Can you work these out from the model? Positions are in its coordinate system, mm. Face numbers are marked on the shaded views. A direction names the side the tool comes from. Coordinates: 2 decimals unless noted, no trailing zeros. Order: outer loops, then holes, each group sorted by start corner. A loop starts at its lowest first (then second) coordinate and runs counter-clockwise, first axis right, second up. Notation, with made-up numbers: (-11, -14) -> (25, -14) arc R17 ccw to (25, -4) -> close; hole circle Ø1 at (-31.75, 55). An arc over 180 degrees is marked (long way). Use a Markdown table: item, result. Add a question column.
1. For pin 1 Ø1.5 at (y, z) = (16.5, 2.5) entering from +X; pin 2 Ø6 at (x, z) = (2, -1) entering from -Y; pin 3 Ø2 at (x, y) = (5.5, 5.5) entering from -Z; pin 4 Ø1.6 at (x, y) = (0, 17.5) entering from -Z, each with a flat end and sliding along its axis, tell me the tip position at first contact or that it passes through.
2. Suppose I cut it at D-D, the plane y = 12.75. List the corners of the cut face in (x, z) for me, then the cut area to 3 significant figures.
3. For the marked faces 4 and 5, which set-ups out of +Z, -Z, +X, -X, +Y, -Y let a thin tool reach every point of the face, with its end or its side?
4. We'd pull the mould along Z, two halves only. Please class the marked faces 1, 2 and 3: pulls with the +Z half, pulls with the -Z half, needs draft (parallel to the pull), parting line crosses it, or undercut.
5. Suppose I cut it at B-B, the plane x = 0. List the corners of the cut face in (y, z) for me.
6. If I drill on line 1 along Z through (x, y) = (0, 4.1); line 2 along X through (y, z) = (17, 0); line 3 along X through (y, z) = (2.75, -0.25), over which ranges is the centre line in solid material (lowest first)? Write a range as from..to.
7. Suppose I cut it at C-C, the plane x = 5.75. List the corners of the cut face in (y, z) for me, then the cut area to 3 significant figures.
8. Suppose I cut it at A-A, the plane y = 3. List the corners of the cut face in (x, z) for me, then the cut area to 3 significant figures.
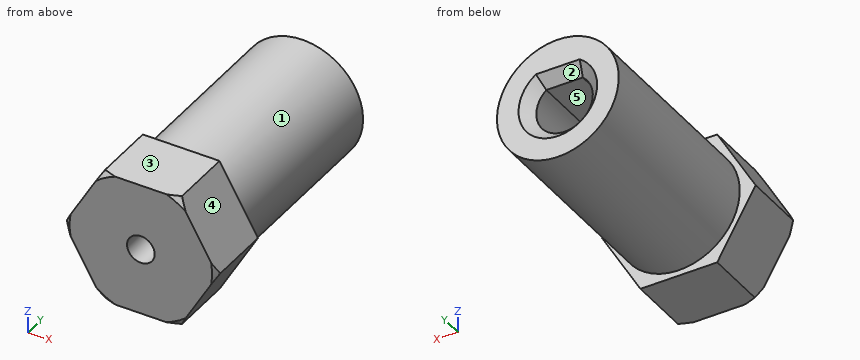
Autodesk Inventor part; units mm, degrees
ref_plane "YZ Plane" through (0, 0, 0) normal (1, 0, 0) x (0, 1, 0)
ref_plane "XZ Plane" through (0, 0, 0) normal (0, 1, 0) x (-1, 0, 0)
ref_plane "XY Plane" through (0, 0, 0) normal (0, 0, 1) x (1, 0, 0)
sketch "Sketch7" plane through (0, 0, 0) normal (0, 1, 0) x (-1, 0, 0)
  line L0 (-3.4641, -6) -> (-6.9282, 0)
  line L1 (-6.9282, 0) -> (-3.4641, 6)
  line L2 (-3.4641, 6) -> (3.4641, 6)
  line L3 (3.4641, 6) -> (6.9282, 0)
  line L4 (6.9282, 0) -> (3.4641, -6)
  line L5 (3.4641, -6) -> (-3.4641, -6)
  point P0 (0, 0)
  point P1 (0, 0)
  point P2 (0, -6)
  dimension "d24" = 12
extrude "Extrusion6" add sketch "Sketch7" along normal blind 6
sketch "Sketch8" plane through (0, 6, 0) normal (0, 1, 0) x (1, 0, 0)
  circle A0 centre (0, 0) radius 5.5
  circle A1 centre (0, 0) radius 2.55
  line L0 (-0.0689, 2.5491) -> (-0.0689, -1.9509)
  line L1 (-0.0689, -1.9509) -> (-1.6421, -1.9509)
  line L2 (-0.0689, -1.9509) -> (1.6421, -1.9509)
  dimension "d27" = 11
  dimension "d28" = 5.1
  dimension "d29" = 4.5
  dimension "d30" = 1.5732
extrude "Extrusion7" add sketch "Sketch8" along normal blind 18 contours A0 | A1 L1 L2
sketch "Sketch9" plane through (0, 0, 0) normal (0, 0, 1) x (1, 0, 0)
  line L0 (6.9282, 0) -> (3.4641, 0)
  line L1 (6.9282, 0) -> (6.4282, 0)
  line L2 (6.8032, 0.3147) -> (6.4282, 0)
  line L3 (6.9282, 0) -> (6.9282, 0.3868)
  line L4 (0, -4.8) -> (0, 28.8)
  line L5 (6.8032, 0.3147) -> (6.9282, 0.4195)
  line L6 (6.9282, 0.4195) -> (6.9282, 0.3868)
  point P0 (0, 0)
  dimension "d33" = 0.5
  dimension "d35" = 40
  dimension "d39" = 0.125
  dimension "d40" = 0.1049
revolve "Revolution1" cut sketch "Sketch9" angle 360 about axis through (0, -10, 0) along (0, 1, 0)
chamfer "Chamfer3" distance 1 angle 45 2 edges at (0, 24, -2.55) (0, 24, 1.9509)
sketch "Sketch10" plane through (0, 0, 0) normal (0, -1, 0) x (1, 0, 0)
  circle A0 centre (0, 0) radius 1.25
  dimension "d44" = 2.5
extrude "Extrusion8" cut sketch "Sketch10" against normal through all
properties part number "PIN_3DPrint"
Worked out:
| question | item | result |
|---|---|---|
| 1 | pin 1 | stops at x = 5.21 |
| 1 | pin 2 | stops at y = 0 |
| 1 | pin 3 | stops at z = -4.21 |
| 1 | pin 4 | stops at z = -5.5 |
| 2 | outline | circle Ø11 at (0, 0); hole (-1.64, 1.95) arc R2.55 ccw (long way) to (1.64, 1.95) -> close |
| 2 | area | 76.0 mm² |
| 3 | face 4 | +Z, +X, +Y, -Y |
| 3 | face 5 | +Y |
| 4 | face 1 | parting line crosses it |
| 4 | face 2 | undercut |
| 4 | face 3 | pulls with the +Z half |
| 5 | outline | (0, -6) -> (6, -6) -> (6, -5.5) -> (24, -5.5) -> (24, -3.55) -> (23, -2.55) -> (6, -2.55) -> (6, -1.25) -> (0, -1.25) -> close; (0, 1.25) -> (6, 1.25) -> (6, 1.95) -> (23, 1.95) -> (24, 2.95) -> (24, 5.5) -> (6, 5.5) -> (6, 6) -> (0, 6) -> close |
| 6 | line 1 | z = -6..-1.25, 1.25..6 |
| 6 | line 2 | x = -5.5..-2.55, 2.55..5.5 |
| 6 | line 3 | x = -6.78..-1.22, 1.22..6.78 |
| 7 | outline | (0, -2.04) -> (6, -2.04) -> (6, 2.04) -> (0, 2.04) -> close |
| 7 | area | 24.5 mm² |
| 8 | outline | (-6.93, 0) -> (-3.46, -6) -> (3.46, -6) -> (6.93, 0) -> (3.46, 6) -> (-3.46, 6) -> close; hole circle Ø2.5 at (0, 0) |
| 8 | area | 120 mm² |
